```python
from build123d import *

# Parameters (mm, degrees)
SKETCH1_W           = 18
SKETCH1_H           = 15
BOSS_EXTRUDE1_DEPTH = 75
SKETCH2_R           = 2.5
CUT_EXTRUDE1_DEPTH  = 12
CUT_EXTRUDE2_DEPTH  = 48
SKETCH4_R           = 2.5
CUT_EXTRUDE3_DEPTH  = 48
FILLET1_R           = 6
BOSS_EXTRUDE2_DEPTH = 10
CHAMFER3_SIZE       = 2
FILLET2_R           = 2
CHAMFER4_SIZE       = 0.25


with BuildPart() as part:
    # Sketch1 → Boss-Extrude1 (new body)
    with BuildSketch(Plane(origin=(0, 0, 0), x_dir=(1, 0, 0), z_dir=(0, 1, 0))):
        with Locations((9, 7.5)):
            Rectangle(SKETCH1_W, SKETCH1_H)
    extrude(amount=BOSS_EXTRUDE1_DEPTH)

    # Sketch2 → Cut-Extrude1 (cut)
    with BuildSketch(Plane.XZ):
        with Locations(Location((14, -6, 0), (0, 0, 270))):
            Circle(SKETCH2_R)
        with Locations(Location((4, -6, 0), (0, 0, 270))):
            Circle(SKETCH2_R)
    extrude(amount=-CUT_EXTRUDE1_DEPTH, mode=Mode.SUBTRACT)

    # Sketch3 → Cut-Extrude2 (cut)
    with BuildSketch(Plane(origin=(18, 0, 0), x_dir=(0, 0, -1), z_dir=(1, 0, 0))):
        Polygon((7.5, 75), (7.5, 29), (15, 21.472065282), (15, 75), align=None)
    extrude(amount=-CUT_EXTRUDE2_DEPTH, mode=Mode.SUBTRACT)

    # Sketch4 → Cut-Extrude3 (cut)
    with BuildSketch(Plane.XY):
        with Locations((9, 70)):
            Circle(SKETCH4_R)
        with Locations((9, 60)):
            Circle(SKETCH4_R)
    extrude(amount=-CUT_EXTRUDE3_DEPTH, mode=Mode.SUBTRACT)

    # Fillet1
    fillet1_edges = [part.edges().sort_by_distance(p)[0] for p in [
        (18, 75, -3.75),
        (0, 75, -3.75),
    ]]
    fillet(fillet1_edges, radius=FILLET1_R)

    # Sketch5 → Boss-Extrude2 (add)
    with BuildSketch(Plane.XZ):
        Polygon((0, 0), (0, 2), (-3, 2), (-3, -18), (21, -18), (21, 2), (18, 2), (18, 0), (18, -15), (0, -15), align=None)
    extrude(amount=-BOSS_EXTRUDE2_DEPTH)

    # Chamfer3
    chamfer3_edges = [part.edges().sort_by_distance(p)[0] for p in [
        (0, 5, 0),
        (18, 5, 0),
    ]]
    chamfer(chamfer3_edges, length=CHAMFER3_SIZE - 0.0001)  # a hair under: the kernel refuses the full size

    # Fillet2
    fillet2_edges = [part.edges().sort_by_distance(p)[0] for p in [
        (21, 5, 2),
        (21, 5, -18),
        (-3, 5, -18),
        (-3, 5, 2),
    ]]
    fillet(fillet2_edges, radius=FILLET2_R)

    # Chamfer4
    chamfer4_edges = [part.edges().sort_by_distance(p)[0] for p in [
        (4, 0, -3.5),
        (14, 0, -3.5),
        (6.5, 70, 0),
        (6.5, 60, 0),
    ]]
    chamfer(chamfer4_edges, length=CHAMFER4_SIZE)


solid = part.part
```
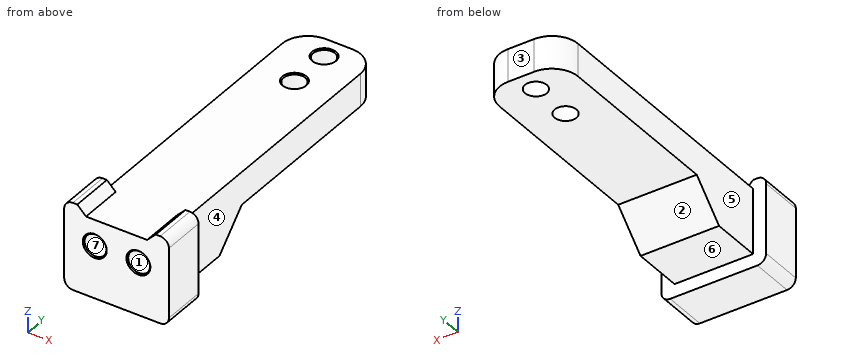
Work out the finished part from the listing and answer in its coordinate system (mm). Face numbers are marked on the shaded views. A direction names the side the tool comes from. Give positions to 0.01 mm unless a question says otherwise; leave off trailing zeros. Write each loop counter-clockwise with the first axis right and the second up, starting at its lowest first coordinate (ties: lowest second). Pieces come first, ordered by that corner, then holes. Notation, with made-up numbers: (74.5, 51.5) -> (80.5, 51.5) arc R22 cw to (80.5, 67.5) -> close; hole circle Ø4 at (27.25, -25). An arc over 180 degrees is marked (long way). Write each question's results on one line, items separated by ' | '.
1. Find section C-C on y = 70. Determine the outline of the cut face in (x, z), and give its area (3 significant figures).
Data:
outline: (0.08, -7.5) -> (6.5, -7.5) -> (6.5, -0.25) -> (6.25, 0) -> (0.08, 0) -> close; (11.5, -7.5) -> (17.92, -7.5) -> (17.92, 0) -> (11.75, 0) -> (11.5, -0.25) -> close | area: 96.2 mm^2
2. Find section D-D on y = 6.5. Give the number of separate pieces and of enclosed holes in the cut face, and give its area (3 significant figures).
Data:
separate pieces: 1 | enclosed holes: 2 | area: 405 mm^2
3. A tool of negligible diameter and unlimited length cuts with its end or side. For the marked faces 4, 5, 6 and 7, from which of +Z, -Z, +X, -X, +Y, -Y can it reach the whole face along a straight path? Write none if from no direction.
Data:
face 4: +Z, -Z, +X, +Y | face 5: +Z, -Z, -X, +Y | face 6: -Z, +X, -X, +Y | face 7: -Y
4. Straight lines are drawn through the part: L1, parallel to X at y = 7.5, z = -6; L2, parallel to Y at x = 10.5, z = -6.25; L3, parallel to Y at x = 10.75, z = -0.25. For each, find the intervals that lie inside material, in ascending order.
Data:
L1: -3 to 1.5, 6.5 to 11.5, 16.5 to 21 | L2: 0 to 58, 62 to 68, 72 to 75 | L3: 0 to 58.21, 61.79 to 68.21, 71.79 to 75
5. Each of these flat-tipped pins is pushed along its axis until it touches: pin 1 Ø1.5 at (x, y) = (11.5, 67.5) entering from +Z; pin 2 Ø4 at (x, y) = (9, 60) entering from -Z; pin 3 Ø2.5 at (x, z) = (15, -6) entering from -Y; pin 4 Ø5.5 at (x, y) = (13, 18) entering from -Z. Where does it stop, or does it pass through?
Data:
pin 1: z = 0 | pin 2: through | pin 3: y = 12 | pin 4: z = -15
6. Find section B-B on z = -6. Determine the outline of the cut face in (x, y).
Data:
outline: (-3, 0) -> (1.25, 0) -> (1.5, 0.25) -> (1.5, 12) -> (6.5, 12) -> (6.5, 0.25) -> (6.75, 0) -> (11.25, 0) -> (11.5, 0.25) -> (11.5, 12) -> (16.5, 12) -> (16.5, 0.25) -> (16.75, 0) -> (21, 0) -> (21, 10) -> (18, 10) -> (18, 69) arc R6 ccw to (12, 75) -> (6, 75) arc R6 ccw to (0, 69) -> (0, 10) -> (-3, 10) -> close; hole circle Ø5 at (9, 60); hole circle Ø5 at (9, 70)
7. Find section A-A on x = 9. Determine the outline of the cut face in (y, z).
Data:
outline: (0, -18) -> (10, -18) -> (10, -15) -> (21.47, -15) -> (29, -7.5) -> (57.5, -7.5) -> (57.5, -0.25) -> (57.25, 0) -> (0, 0) -> close; (62.5, -7.5) -> (67.5, -7.5) -> (67.5, -0.25) -> (67.25, 0) -> (62.75, 0) -> (62.5, -0.25) -> close; (72.5, -7.5) -> (75, -7.5) -> (75, 0) -> (72.75, 0) -> (72.5, -0.25) -> close
8. Determine the mould class of the marked faces 1, 2 and 3 for opening direction Z: +Z half, -Z half, draft (parallel to the pull), parting line (faces both ways), or undercut.
Data:
face 1: undercut | face 2: -Z half | face 3: draft
